Here's how the part is built. I have some questions about the finished solid (model axes, mm). A direction names the side the tool comes from. Round coordinates to 2 decimals unless told otherwise and drop trailing zeros. Order: outer loops, then holes, each group sorted by start corner. A loop starts at its lowest first (then second) coordinate and runs counter-clockwise, first axis right, second up. Notation, with made-up numbers: (-28.5, 46) -> (5.5, 46) arc R9 ccw to (5.5, 51) -> close; hole circle Ø1 at (-20.5, 25). An arc over 180 degrees is marked (long way). One line per item, written item: value.
```python
from build123d import *
from build123d import SkipClean  # not in build123d's __all__

# Parameters (mm, degrees)
F3_DEPTH      = 25
F3_DEPTH_BACK = 25
F6_DEPTH      = 10
F6_DEPTH_BACK = 10
F7_SIZE       = 1


with BuildPart() as f1:
    # F0 (on Front) → F1 (revolve)
    with BuildSketch(Plane.XZ):
        Polygon((-12.5, 11.5), (-15, 11.5), (-15, 0), (-15, -11.5), (-12.5, -11.5), (-12.5, -25), (-10, -25), (-10, -45), (0, -45), (0, 0), (0, 45), (-10, 45), (-10, 25), (-12.5, 25), align=None)
    revolve(axis=Axis((0, 0, 22.5), (0, 0, -1)))

    # F2 (on Top) → F3 (cut, two sides)
    with BuildSketch(Plane.XY) as f3_sk:
        Polygon((0, -13), (-15, -13), (-15, -17), (0, -17), (15, -17), (15, -13), align=None)
    extrude(amount=F3_DEPTH, mode=Mode.SUBTRACT)
    extrude(f3_sk.sketch, amount=-F3_DEPTH_BACK, mode=Mode.SUBTRACT)

    # F5 (on offset) → F6 (join, two sides)
    with BuildSketch(Plane.XY.offset(45)) as f6_sk:
        with BuildLine():
            Line((9.6824583655, 2.5), (-9.6824583655, 2.5))
            ThreePointArc((-9.6824583655, 2.5), (-10, 0), (-9.6824583655, -2.5))
            Line((-9.6824583655, -2.5), (9.6824583655, -2.5))
            ThreePointArc((9.6824583655, -2.5), (10, 0), (9.6824583655, 2.5))
        make_face()
    with SkipClean():  # cleaning this boolean's faces spoils the solid; the shape is the same uncleaned
        extrude(amount=F6_DEPTH)
        extrude(f6_sk.sketch, amount=-F6_DEPTH_BACK)

    # F7
    f7_edges = [f1.edges().sort_by_distance(p)[0] for p in [
        (10, 0, 55),
        (-10, 0, 55),
    ]]
    chamfer(f7_edges, length=F7_SIZE)


solid = f1.part
```
Q1. I want a section at D-D on x = 6. Write out the boundary of the cut face in (y, z), then the cut area to 3 significant figures.
Answers:
outline: (-13, -11.5) -> (-10.97, -11.5) -> (-10.97, -25) -> (-8, -25) -> (-8, -45) -> (8, -45) -> (8, -25) -> (10.97, -25) -> (10.97, -11.5) -> (13.75, -11.5) -> (13.75, 11.5) -> (10.97, 11.5) -> (10.97, 25) -> (8, 25) -> (8, 45) -> (2.5, 45) -> (2.5, 55) -> (-2.5, 55) -> (-2.5, 45) -> (-8, 45) -> (-8, 25) -> (-10.97, 25) -> (-10.97, 11.5) -> (-13, 11.5) -> close
area: 1,900 mm2
Q2. For P1, Ø1.5, axis at y = -5, z = -16, coming from the -X side; P2, Ø5, axis at x = -1, z = 51.5, coming from the -Y side; P3, Ø2, axis at x = -12, y = -3, coming from the -Z side; P4, Ø5, axis at y = 2.5, z = 0, coming from the +X side, each with a flat end and sliding along its axis, tell me the tip position at first contact or that it passes through.
Answers:
P1: x = -11.76
P2: y = -2.5
P3: z = -25
P4: x = 15
Q3. I want a section at C-C on y = 8. Write out the boundary of the cut face in (x, z), then the cut area to 3 significant figures.
Answers:
outline: (-12.69, -11.5) -> (-9.6, -11.5) -> (-9.6, -25) -> (-6, -25) -> (-6, -45) -> (6, -45) -> (6, -25) -> (9.6, -25) -> (9.6, -11.5) -> (12.69, -11.5) -> (12.69, 11.5) -> (9.6, 11.5) -> (9.6, 25) -> (6, 25) -> (6, 45) -> (-6, 45) -> (-6, 25) -> (-9.6, 25) -> (-9.6, 11.5) -> (-12.69, 11.5) -> close
area: 1,580 mm2
Q4. I want a section at B-B on z = 41. Write out the boundary of the cut face in (x, y), then the cut area to 3 significant figures.
Answers:
outline: circle Ø20 at (0, 0)
area: 314 mm2
Q5. Which directions (+Z, -Z, +X, -X, +Y, -Y) give clear straight access to the entire face, cutting with the end or side of a thin tool? Please do faces 1 (the face through (0, -2.5, 50)), 2 (the face through (2.17, -9.76, -35.14)), 3 (the face through (2.2, 12.5, 11.5)).
Answers:
face 1: +Z, +X, -X, -Y
face 2: -Z
face 3: +Z
Q6. I need wall thicknesses on line 1 along Z through (x, y) = (-0.25, 13); line 2 along Y through (x, z) = (-13, 8); line 3 along Z through (x, y) = (7.5, 5.25). Which ranges of each line are inside material? Lowest first, please.
Answers:
line 1: -11.5 to 11.5
line 2: -7.48 to 7.48
line 3: -45 to 45
Q7. I want a section at A-A on x = 0. Write out the boundary of the cut face in (y, z).
Answers:
outline: (-13, -11.5) -> (-12.5, -11.5) -> (-12.5, -25) -> (-10, -25) -> (-10, -45) -> (10, -45) -> (10, -25) -> (12.5, -25) -> (12.5, -11.5) -> (15, -11.5) -> (15, 11.5) -> (12.5, 11.5) -> (12.5, 25) -> (10, 25) -> (10, 45) -> (2.5, 45) -> (2.5, 55) -> (-2.5, 55) -> (-2.5, 45) -> (-10, 45) -> (-10, 25) -> (-12.5, 25) -> (-12.5, 11.5) -> (-13, 11.5) -> close
